Check sheet for the modelled part. Datum: model origin and axes. Units: mm. A direction names the side the tool comes from. Round coordinates to 2 decimals unless told otherwise and drop trailing zeros. Write each loop counter-clockwise with the first axis right and the second up, starting at its lowest first coordinate (ties: lowest second). Pieces come first, ordered by that corner, then holes. Notation, with made-up numbers: (-27.75, -39) -> (-11.75, -39) arc R11 cw to (-11.75, -26) -> close; hole circle Ø2 at (76.5, 62.5). An arc over 180 degrees is marked (long way). One line per item, written item: value.
Autodesk Inventor part; units mm, degrees
ref_plane "YZ Plane" through (0, 0, 0) normal (1, 0, 0) x (0, 1, 0)
ref_plane "XZ Plane" through (0, 0, 0) normal (0, 1, 0) x (-1, 0, 0)
ref_plane "XY Plane" through (0, 0, 0) normal (0, 0, 1) x (1, 0, 0)
sketch "Sketch1" plane through (0, 0, 0) normal (0, 1, 0) x (-1, 0, 0)
  circle A0 centre (0, 0) radius 6.86
  dimension "d0" = 13.72
extrude "Extrusion1" add sketch "Sketch1" along normal blind 1.5
sketch "Sketch2" plane through (0, 1.5, 0) normal (0, 1, 0) x (1, 0, 0)
  line L0 (-2.3452, -5.25) -> (2.3452, -5.25)
  line L1 (2.3452, 5.25) -> (-2.3452, 5.25)
  line L2 (0, 0) -> (0, 5.25) construction
  line L3 (0, 0) -> (0, -5.25) construction
  arc A0 (2.3452, -5.25) -> (2.3452, 5.25) centre (0, 0) ccw
  arc A1 (-2.3452, 5.25) -> (-2.3452, -5.25) centre (0, 0) ccw
  dimension "Barrel_Flat_Width" = 10.5
  dimension "d5" = 5.75
extrude "Extrusion2" add sketch "Sketch2" along normal blind 10.86
thread "Thread1"
thread "Thread2"
sketch "Sketch3" plane through (0, 0, 0) normal (0, -1, 0) x (1, 0, 0)
  circle A0 centre (1.81, 0) radius 3.05
  line L0 (0, 0) -> (1.81, 0) construction
  circle A1 centre (0, 0) radius 6.86 construction
  dimension "d12" = 6.1
  dimension "d14" = 2
extrude "Extrusion3" cut sketch "Sketch3" against normal blind 9
sketch "Sketch4" plane through (1.81, 9, 0) normal (0, -1, 0) x (1, 0, 0)
  circle A0 centre (0, 0) radius 3.05 construction
  circle A1 centre (0, 0) radius 1.05
  point P0 (-1.81, 0)
  dimension "d17" = 2.1
extrude "Extrusion4" add sketch "Sketch4" along normal blind 7.83
fillet "Fillet1" radius 1.05 1 edges at (0.76, 1.17, 0)
properties part number "Barrel_Jack" material "PC/ABS Plastic"
Item 1: Sectioned sample at C-C on x = 3.25. Enter the section's corners in (y, z).
Answer:
outline: (0, -6.04) -> (1.5, -6.04) -> (1.5, -4.74) -> (12.36, -4.74) -> (12.36, 4.74) -> (1.5, 4.74) -> (1.5, 6.04) -> (0, 6.04) -> (0, 2.69) -> (9, 2.69) -> (9, -2.69) -> (0, -2.69) -> close
Item 2: Depth check by flat-ended pin: P1, Ø2.5, axis at x = 1, y = 6.5, coming from the -Z side; P2, Ø1.5, axis at x = 5, y = 7.5, coming from the +Z side; P3, Ø3, axis at y = 9, z = 1, coming from the +X side. Enter the tip coordinate at first touch or a pass-through.
Answer:
P1: stops at z = -5.25
P2: stops at z = 3.87
P3: stops at x = 5.75
Item 3: Sectioned sample at A-A on y = 3. Enter the section's corners in (x, z).
Answer:
outline: (-2.35, -5.25) -> (2.35, -5.25) arc R5.75 ccw to (2.35, 5.25) -> (-2.35, 5.25) arc R5.75 ccw to start; circle Ø2.1 at (1.81, 0); hole circle Ø6.1 at (1.81, 0)
Item 4: Tool access check on faces 4 (the cylindrical face through (4.72, 4.44, 0.92)), 5 (the flat face through (0, 1.5, 6)), 6 (the flat face through (0, 7, -5.25)), 7 (the cylindrical face through (-5.75, 6.85, 0.09)). Record the directions out of +Z, -Z, +X, -X, +Y, -Y that give a thin tool (end or side, any length) a straight path to the whole face; none if there is none.
Answer:
face 4: -Y
face 5: +Y
face 6: -Z, +X, -X, +Y
face 7: -X, +Y
Item 5: Sectioned sample at B-B on z = 0. Enter the section's corners in (x, y), and give its area (3 significant figures).
Answer:
outline: (-6.86, 0) -> (-1.24, 0) -> (-1.24, 9) -> (0.76, 9) -> (0.76, 2.22) arc R1.05 ccw to (2.86, 2.22) -> (2.86, 9) -> (4.86, 9) -> (4.86, 0) -> (6.86, 0) -> (6.86, 1.5) -> (5.75, 1.5) -> (5.75, 12.36) -> (-5.75, 12.36) -> (-5.75, 1.5) -> (-6.86, 1.5) -> close
area: 107 mm^2
Item 6: Sectioned sample at D-D on z = 2.5. Enter the section's corners in (x, y).
Answer:
outline: (-6.39, 0) -> (0.06, 0) -> (0.06, 9) -> (3.56, 9) -> (3.56, 0) -> (6.39, 0) -> (6.39, 1.5) -> (5.18, 1.5) -> (5.18, 12.36) -> (-5.18, 12.36) -> (-5.18, 1.5) -> (-6.39, 1.5) -> close
Item 7: Mould release check, pull along Z, two halves, no side actions. Record for faces 1 (the flat face through (3.1, 9, 0)), 2 (the cylindrical face through (5.75, 6.85, -0.09)), 3 (the flat face through (-1.4, 0, 0.1)): pulls with the +Z half, pulls with the -Z half, needs draft (parallel to the pull), parting line crosses it, or undercut.
Answer:
face 1: undercut
face 2: parting line crosses it
face 3: needs draft
Item 8: Thickness scan on line 1 (Z direction, x = 1.81, y = 7.25); line 2 (Y direction, x = 3, z = 1); line 3 (Z direction, x = -5.25, y = 6.75). Record the ranges inside material, lowest first.
Answer:
line 1: z = -5.25 to -3.05, -1.05 to 1.05, 3.05 to 5.25
line 2: y = 9 to 12.36
line 3: z = -2.35 to 2.35
